Model file for the job. Use its own axes, mm. Face numbers are marked on the shaded views. Give positions to 0.01 mm unless a question says otherwise; leave off trailing zeros. Write each loop counter-clockwise with the first axis right and the second up, starting at its lowest first coordinate (ties: lowest second). Pieces come first, ordered by that corner, then holes. Notation, with made-up numbers: M -25.5,42.25 L -20.5,42.25 A21 ccw -20.5,54.25 Z; hole C -27.75,-22.75 d11. An arc over 180 degrees is marked long. Answer as a JSON object with one key per item and string values. Group by question number.
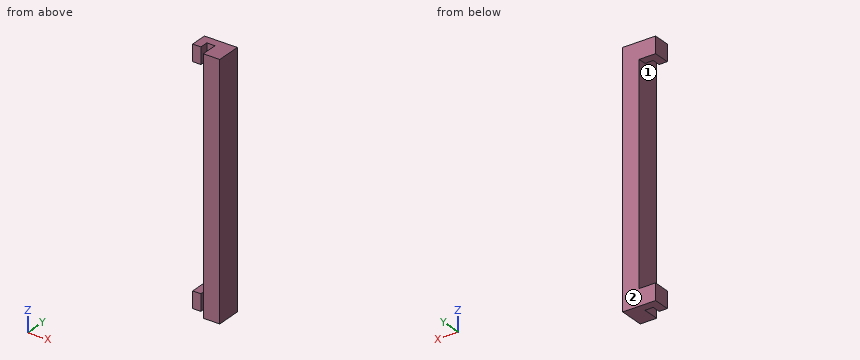
```python
from build123d import *

# Parameters (mm, degrees)
BOSS_EXTRUDE1_DEPTH     = 30
CUT_EXTRUDE1_DEPTH      = 1
CUT_EXTRUDE1_DEPTH_BACK = 301


with BuildPart() as part:
    # Sketch3 → Boss-Extrude1 (new body)
    with BuildSketch(Plane(origin=(0, 0, 0), x_dir=(1, 0, 0), z_dir=(0, 1, 0))):
        Polygon((0, 0), (0, 20), (40, 20), (40, -280), (0, -280), (0, -260), (20, -260), (20, 0), align=None)
    extrude(amount=BOSS_EXTRUDE1_DEPTH)

    # Sketch4 → Cut-Extrude1 (cut, two sides)
    with BuildSketch(Plane.XY.offset(280)) as cut_extrude1_sk:
        Polygon((0, 10), (10, 10), (10, 20), (20, 20), (20, 0), (0, 0), align=None)
    extrude(amount=CUT_EXTRUDE1_DEPTH, mode=Mode.SUBTRACT)
    extrude(cut_extrude1_sk.sketch, amount=-CUT_EXTRUDE1_DEPTH_BACK, mode=Mode.SUBTRACT)


solid = part.part
```
Q1. Two-plate mould, pull along Z, no slides. Class the marked faces 1 and 2: +Z half, -Z half, draft (parallel to the pull), parting line (faces both ways), or undercut.
Q2. Slice it at B-B, the plane y = 17.25. Write the cut outline in (x, z), then the cut area to 3 significant figures.
Q3. Slice it at D-D, the plane z = 9.5. Write the cut outline in (x, y).
Q4. Slice it at A-A, the plane x = 7. Write the cut outline in (y, z).
Q5. Slice it at C-C, the plane y = 4.75. Write the cut outline in (x, z).
Q6. Wall check: L1, parallel to Z at x = 7, y = 26.75; L2, parallel to X at y = 7.5, z = 219.5. Give the ranges that are in metal, low to high.
Q7. Drop flat-ended pins along their axis: P1, Ø4, axis at y = 13.5, z = 169, coming from the -X side; P2, Ø11, axis at x = 5, z = 266, coming from the -Y side; P3, Ø5, axis at x = 15.5, z = 272.5, coming from the -Y side. Give the stop position or say it passes through.
Solved:
{
 "1": {"face 1": "undercut", "face 2": "draft"},
 "2": {"outline": "M 0,-20 L 10,-20 L 10,0 L 0,0 Z; M 0,260 L 10,260 L 10,280 L 0,280 Z; M 20,-20 L 40,-20 L 40,280 L 20,280 Z", "area": "6,400 mm²"},
 "3": {"outline": "M 20,0 L 40,0 L 40,30 L 20,30 Z"},
 "4": {"outline": "M 10,-20 L 30,-20 L 30,0 L 10,0 Z; M 10,260 L 30,260 L 30,280 L 10,280 Z"},
 "5": {"outline": "M 20,-20 L 40,-20 L 40,280 L 20,280 Z"},
 "6": {"L1": "z = -20 to 0, 260 to 280", "L2": "x = 20 to 40"},
 "7": {"P1": "stops at x = 20", "P2": "stops at y = 10", "P3": "stops at y = 20"}
}
